```python
from build123d import *

# Parameters (mm, degrees)
F0_W     = 31.956
F0_H     = 15.78
F0_W_2   = 28.842
F0_H_2   = 13.12
F1_DEPTH = 9.6
F2_DEPTH = 25
F3_DEPTH = 1.557
F4_R     = 3.267
F4_R_2   = 2.467
F5_DEPTH = 8.043
F6_R     = 2.45
F7_DEPTH = 2.1


with BuildPart() as f1:
    # F0 (on Top) → F1 (new body)
    with BuildSketch(Plane.XY):
        with Locations((-20.927882, -12.640023)):
            Rectangle(F0_W, F0_H)
        with Locations((-20.927882, -12.640023)):
            Rectangle(F0_W_2, F0_H_2, mode=Mode.SUBTRACT)
        with Locations((-20.927882, -12.640023)):
            Rectangle(F0_W_2, F0_H_2)
    extrude(amount=F1_DEPTH)

    # F0 (on Top) → F2 (cut)
    with BuildSketch(Plane.XY):
        with Locations((-20.927882, -12.640023)):
            Rectangle(F0_W_2, F0_H_2)
    extrude(amount=F2_DEPTH, mode=Mode.SUBTRACT)

    # F0 (on Top) → F3 (join)
    with BuildSketch(Plane.XY):
        with Locations((-20.927882, -12.640023)):
            Rectangle(F0_W_2, F0_H_2)
    extrude(amount=F3_DEPTH)

    # F4 (on face) → F5 (join)
    with BuildSketch(Plane.XY.offset(1.557)):
        with Locations((-28.941882, -12.714023)):
            Circle(F4_R)
        with Locations((-28.941882, -12.714023)):
            Circle(F4_R_2, mode=Mode.SUBTRACT)
        with Locations((-20.927882, -12.714023)):
            Circle(F4_R)
        with Locations((-20.927882, -12.714023)):
            Circle(F4_R_2, mode=Mode.SUBTRACT)
        with Locations((-12.913882, -12.714023)):
            Circle(F4_R)
        with Locations((-12.913882, -12.714023)):
            Circle(F4_R_2, mode=Mode.SUBTRACT)
    extrude(amount=F5_DEPTH)

    # F6 (on face) → F7 (join)
    with BuildSketch(Plane(origin=(0, 0, 0), x_dir=(1, 0, 0), z_dir=(0, 0, -1))):
        with Locations((-32.948882, 16.573023)):
            Circle(F6_R)
        with Locations((-24.844882, 16.573023)):
            Circle(F6_R)
        with Locations((-16.740882, 16.573023)):
            Circle(F6_R)
        with Locations((-8.636882, 16.573023)):
            Circle(F6_R)
        with Locations((-8.636882, 8.707023)):
            Circle(F6_R)
        with Locations((-16.740882, 8.707023)):
            Circle(F6_R)
        with Locations((-24.844882, 8.707023)):
            Circle(F6_R)
        with Locations((-32.948882, 8.707023)):
            Circle(F6_R)
    extrude(amount=F7_DEPTH)


solid = f1.part
```
Model file for the job. Use its own axes, mm. A direction names the side the tool comes from. Coordinates: 2 decimals unless noted, no trailing zeros. Write each loop counter-clockwise with the first axis right and the second up, starting at its lowest first coordinate (ties: lowest second). Pieces come first, ordered by that corner, then holes. Notation, with made-up numbers: (60.5, -13.5) - (119.5, -13.5) arc R21 ccw to (119.5, -4.5) - close; hole circle Ø3 at (52, 6). An arc over 180 degrees is marked (long way). One line per question, with ' | ' between items. Start each with the question number.
Q1. Cut at C-C, the plane x = -22. List the corners of the cut face in (y, z).
Q2. Pull direction X, two halves, no side cores. Call faces 1 (the face through (-4.95, -13, 5)), 2 (the face through (-33, -9, -2.1)), 3 (the face through (-29, -13, 1.557)): pulls with the +X half, pulls with the -X half, needs draft (parallel to the pull), parting line crosses it, or undercut.
Q3. 3-axis set-ups, long thin cutter, end or side, ignore diameter. For faces 4 (the face through (-17, -17, -2.1)), 5 (the face through (-8.96, -19, -1.04)), 6 (the face through (-13.339, -9.475, 5.522)): which of +Z, -Z, +X, -X, +Y, -Y reach the whole face in a straight line?
Q4. Cut at B-B, the plane z = 3.25. List the corners of the cut face in (x, y).
Q5. Pin check, flat tips, straight feed: pin 1 (1.5 mm diameter, centred on x = -22.5, y = -7.5, fed in from +Z); pin 2 (5.5 mm diameter, centred on x = -12.91, y = -12.71, fed in from -Z); pin 3 (6 mm diameter, centred on x = -13.5, y = -12, fed in from -Z). Stop position of each tip, or through.
Q6. Cut at A-A, the plane z = -1.5. List the corners of the cut face in (x, y).
Q7. Drill centre lines: line 1 (X direction, y = -7.5, z = 7.25); line 2 (Y direction, x = -8, z = 7.25); line 3 (X direction, y = -9, z = -0.5). Where is each one in solid material? Low to high. Write a range as [from, to].
Q8. Cut at D-D, the plane y = -6.75. List the corners of the cut face in (x, z).
Answer below:
1) outline: (-20.53, 0) - (-4.75, 0) - (-4.75, 9.6) - (-6.08, 9.6) - (-6.08, 1.56) - (-9.63, 1.56) - (-9.63, 9.6) - (-10.49, 9.6) - (-10.49, 1.56) - (-14.94, 1.56) - (-14.94, 9.6) - (-15.8, 9.6) - (-15.8, 1.56) - (-19.2, 1.56) - (-19.2, 9.6) - (-20.53, 9.6) - close
2) face 1: pulls with the +X half | face 2: needs draft | face 3: undercut
3) face 4: -Z, +X, -X, +Y, -Y | face 5: -Z | face 6: +Z
4) outline: (-36.91, -20.53) - (-4.95, -20.53) - (-4.95, -4.75) - (-36.91, -4.75) - close; circle Ø6.53 at (-28.94, -12.71); circle Ø6.53 at (-20.93, -12.71); circle Ø6.53 at (-12.91, -12.71); hole (-35.35, -19.2) - (-6.51, -19.2) - (-6.51, -6.08) - (-35.35, -6.08) - close; hole circle Ø4.93 at (-28.94, -12.71); hole circle Ø4.93 at (-20.93, -12.71); hole circle Ø4.93 at (-12.91, -12.71)
5) pin 1: z = 1.56 | pin 2: z = 0 | pin 3: z = -2.1
6) outline: circle Ø4.9 at (-32.95, -16.57); circle Ø4.9 at (-32.95, -8.71); circle Ø4.9 at (-24.84, -16.57); circle Ø4.9 at (-24.84, -8.71); circle Ø4.9 at (-16.74, -16.57); circle Ø4.9 at (-16.74, -8.71); circle Ø4.9 at (-8.64, -16.57); circle Ø4.9 at (-8.64, -8.71)
7) line 1: [-36.91, -35.35], [-6.51, -4.95] | line 2: [-20.53, -19.2], [-6.08, -4.75] | line 3: [-35.38, -30.52], [-27.28, -22.41], [-19.17, -14.31], [-11.07, -6.2]
8) outline: (-36.91, 0) - (-34.42, 0) - (-34.42, -2.1) - (-31.47, -2.1) - (-31.47, 0) - (-26.32, 0) - (-26.32, -2.1) - (-23.37, -2.1) - (-23.37, 0) - (-18.21, 0) - (-18.21, -2.1) - (-15.27, -2.1) - (-15.27, 0) - (-10.11, 0) - (-10.11, -2.1) - (-7.16, -2.1) - (-7.16, 0) - (-4.95, 0) - (-4.95, 9.6) - (-6.51, 9.6) - (-6.51, 1.56) - (-35.35, 1.56) - (-35.35, 9.6) - (-36.91, 9.6) - close
